Design review of the part built by this model. Coordinates are the model's own, in mm. A direction names the side the tool comes from. Coordinates: 2 decimals unless noted, no trailing zeros. Loops run counter-clockwise (first coordinate to the right, second up) from the corner with the lowest first, then second, coordinate; pieces in that order, holes last. Notation, with made-up numbers: (60.5, 69) -> (96.5, 69) arc R9 cw to (96.5, 80) -> close; hole circle Ø11 at (87, 72). An arc over 180 degrees is marked (long way). Use CSV: the item, a comma, the result in double quotes.
Autodesk Inventor part; units mm, degrees
ref_plane "YZ Plane" through (0, 0, 0) normal (1, 0, 0) x (0, 1, 0)
ref_plane "XZ Plane" through (0, 0, 0) normal (0, 1, 0) x (-1, 0, 0)
ref_plane "XY Plane" through (0, 0, 0) normal (0, 0, 1) x (1, 0, 0)
sketch "Sketch1" plane through (0, 0, 0) normal (1, 0, 0) x (0, 1, 0)
  line L0 (12.7, 12.2788) -> (-12.7, 12.2788)
  line L1 (-12.7, 12.2788) -> (-12.7, -13.1212)
  line L2 (-12.7, -13.1212) -> (12.7, -13.1212)
  line L3 (12.7, -13.1212) -> (12.7, 12.2788)
  line L4 (0, 32.4321) -> (0, -31.5519)
  line L5 (24.3369, 0) -> (-19.9975, 0)
  line L6 (11.1125, -11.5337) -> (-11.1125, -11.5337)
  line L7 (-11.1125, -11.5337) -> (-11.1125, 10.6913)
  line L8 (-11.1125, 10.6913) -> (11.1125, 10.6913)
  line L9 (11.1125, 10.6913) -> (11.1125, -11.5337)
  point P0 (0, 0)
  dimension "d0" = 25.4
  dimension "d24" = 1.5875
  dimension "d25" = 1.5875
  dimension "d26" = 1.5875
  dimension "d27" = 1.5875
extrude "Extrusion1" add sketch "Sketch1" along normal blind 342.9 contours L3 L5 L9 L8 L4 L0 | L4 L8 L7 L5 L1 L0 | L3 L2 L4 L6 L9 L5 | L5 L7 L6 L4 L2 L1
equation "\"d25\" = d24"
equation "\"d26\" = d24"
equation "\"d27\" = d26"
properties part number "Part1-17-13.31255in" material "Aluminum 6061"
Item 1: Draft analysis for pull direction Y (two halves, no side actions). For faces 3 (the face through (169, -11.112, -1)), 4 (the face through (0, -11.3, -0.4)), 5 (the face through (169, 12.7, -1)), state which applies: pulls with the +Y half, pulls with the -Y half, needs draft (parallel to the pull), parting line crosses it, or undercut.
Checked values:
face 3,"undercut"
face 4,"needs draft"
face 5,"pulls with the +Y half"
Item 2: Machinability: for faces 1 (the face through (169, 0, 10.691)), 2 (the face through (342.9, -11.3, -0.4)), which of the approach directions +Z, -Z, +X, -X, +Y, -Y give a long, thin tool a straight path to every point of the face, cutting with its end or side? Answer none if there is none.
Checked values:
face 1,"+X, -X"
face 2,"+Z, -Z, +X, +Y, -Y"
Item 3: To check wall thickness, follow line 1 along Y through (x, z) = (177, 3.5); line 2 along Z through (x, y) = (189.5, 6). State the ranges of each line that lie inside material, in increasing order.
Checked values:
line 1,"-12.7 to -11.11, 11.11 to 12.7"
line 2,"-13.12 to -11.53, 10.69 to 12.28"
Item 4: Add section A-A (z = -2.5). Give the boundary of the cut face in (x, y).
Checked values:
outline,"(0, -12.7) -> (342.9, -12.7) -> (342.9, -11.11) -> (0, -11.11) -> close; (0, 11.11) -> (342.9, 11.11) -> (342.9, 12.7) -> (0, 12.7) -> close"
Item 5: Add section B-B (y = -2.5). Give the boundary of the cut face in (x, z), then the cut area to 3 significant figures.
Checked values:
outline,"(0, -13.12) -> (342.9, -13.12) -> (342.9, -11.53) -> (0, -11.53) -> close; (0, 10.69) -> (342.9, 10.69) -> (342.9, 12.28) -> (0, 12.28) -> close"
area,"1,090 mm^2"
Item 6: Add section C-C (x = 202). Give the boundary of the cut face in (y, z).
Checked values:
outline,"(-12.7, -13.12) -> (12.7, -13.12) -> (12.7, 12.28) -> (-12.7, 12.28) -> close; hole (-11.11, -11.53) -> (11.11, -11.53) -> (11.11, 10.69) -> (-11.11, 10.69) -> close"
